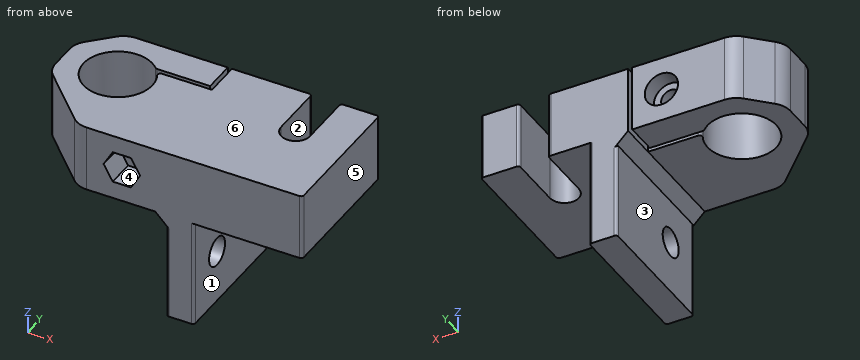
```python
from build123d import *

# Parameters (mm, degrees)
PAD_DEPTH       = 31.5
SKETCH001_W     = 20
SKETCH001_H     = 30
SKETCH001_W_2   = 27
POCKET_DEPTH    = 19.5
SKETCH002_R     = 2.6
POCKET001_DEPTH = 24.501
SKETCH003_R     = 1.7
POCKET002_DEPTH = 25.001
SKETCH004_R     = 3
POCKET003_DEPTH = 3
POCKET004_DEPTH = 5
CHAMFER_SIZE    = 2
FILLET_R        = 0.5


with BuildPart() as body:
    # Sketch → Pad (new body)
    with BuildSketch(Plane.XY):
        with BuildLine():
            ThreePointArc((-0.171573, -13.828427), (1.126121, -14.695518), (2.656854, -15))
            Line((41.00007, -14.999422), (2.656854, -15))
            ThreePointArc((41.00007, -14.999422), (41.353579, -14.85295), (41.5, -14.499421))
            Line((41.5, 9.5), (41.5, -14.499421))
            ThreePointArc((41.5, 9.5), (41.353578, 9.853528), (41.000071, 10))
            Line((34.6, 10), (41.000071, 10))
            Line((34.6, 10), (34.6, 0))
            ThreePointArc((29.4, 0), (32, -2.6), (34.6, 0))
            Line((29.4, 0), (29.4, 10))
            Line((15, 10), (29.4, 10))
            Line((15, 3.5), (15, 10))
            Line((5.990826, 3.5), (15, 3.5))
            ThreePointArc((5.990826, 3.5), (5.56542, 3.262735), (5.54375, 2.776119))
            ThreePointArc((4.372572, 4.395522), (-5.023841, -3.633322), (5.54375, 2.776119))
            ThreePointArc((4.372572, 4.395522), (4.534461, 4.28781), (4.725198, 4.25))
            Line((14.25, 4.25), (4.725198, 4.25))
            Line((14.25, 10), (14.25, 4.25))
            Line((-2.343146, 10), (14.25, 10))
            ThreePointArc((-2.343146, 10), (-3.873879, 9.695518), (-5.171573, 8.828427))
            Line((-5.171573, 8.828427), (-8.828427, 5.171573))
            ThreePointArc((-8.828427, 5.171573), (-9.695518, 3.873879), (-10, 2.343146))
            Line((-10, -2.343146), (-10, 2.343146))
            ThreePointArc((-10, -2.343146), (-9.695518, -3.873879), (-8.828427, -5.171573))
            Line((-8.828427, -5.171573), (-0.171573, -13.828427))
        make_face()
    extrude(amount=PAD_DEPTH)

    # Sketch001 (on Face26 of Pad) → Pocket (cut)
    with BuildSketch(Plane.XY.offset(31.5)):
        with Locations((32, 0)):
            Rectangle(SKETCH001_W, SKETCH001_H)
        with Locations((3.5, 0)):
            Rectangle(SKETCH001_W_2, SKETCH001_H)
    extrude(amount=-POCKET_DEPTH, mode=Mode.SUBTRACT)

    # Sketch002 (on Face29 of Pocket) → Pocket001 (cut, through all)
    with BuildSketch(Plane(origin=(17, 0, 0), x_dir=(0, -1, 0), z_dir=(-1, 0, 0))):
        with Locations((7.5, 22)):
            Circle(SKETCH002_R)
    extrude(amount=-POCKET001_DEPTH, mode=Mode.SUBTRACT)

    # Sketch003 (on Face13 of Pocket001) → Pocket002 (cut, through all)
    with BuildSketch(Plane(origin=(0, 10, 0), x_dir=(-1, 0, 0), z_dir=(0, 1, 0))):
        with Locations((-9, 6)):
            Circle(SKETCH003_R)
    extrude(amount=-POCKET002_DEPTH, mode=Mode.SUBTRACT)

    # Sketch004 (on Face13 of Pocket002) → Pocket003 (cut)
    with BuildSketch(Plane(origin=(0, 10, 0), x_dir=(-1, 0, 0), z_dir=(0, 1, 0))):
        with Locations((-9, 6)):
            Circle(SKETCH004_R)
    extrude(amount=-POCKET003_DEPTH, mode=Mode.SUBTRACT)

    # Sketch005 (on Face21 of Pocket003) → Pocket004 (cut)
    with BuildSketch(Plane(origin=(0.000226, -15.00004, 0), x_dir=(1, 1.5e-05, 0), z_dir=(1.5e-05, -1, 0))):
        Polygon((10.645448, 3.15), (12.290897, 6), (10.645448, 8.85), (7.354552, 8.85), (5.709103, 6), (7.354552, 3.15), align=None)
    extrude(amount=-POCKET004_DEPTH, mode=Mode.SUBTRACT)

    # Chamfer
    chamfer_edges = [body.edges().sort_by_distance(p)[0] for p in [
        (17, -2.499892, 12),
    ]]
    chamfer(chamfer_edges, length=CHAMFER_SIZE)

    # Fillet
    fillet_edges = [body.edges().sort_by_distance(p)[0] for p in [
        (34.6, 10, 6),
        (29.4, 10, 6),
        (22, 10, 21.75),
        (22, -14.999708, 21.75),
        (17, 10, 22.75),
        (17, -14.999784, 22.75),
    ]]
    fillet(fillet_edges, radius=FILLET_R)


with BuildPart() as part_mirroring:
    # Part__Mirroring: instance of Body
    add(body.part.mirror(Plane(origin=(15.75, -2.5, 0), x_dir=(0, 1, 0), z_dir=(0, 0, 1))))


solid = part_mirroring.part
```
The listing builds one solid part. Answer for the finished solid, in the listing's coordinates (mm). Face numbers are marked on the shaded views. A direction names the side the tool comes from. Round coordinates to 2 decimals unless told otherwise and drop trailing zeros. Order: outer loops, then holes, each group sorted by start corner. A loop starts at its lowest first (then second) coordinate and runs counter-clockwise, first axis right, second up. Notation, with made-up numbers: (-22.5, -3.5) - (3.5, -3.5) arc R26 ccw to (3.5, 26.5) - close; hole circle Ø7 at (-35, 61.5). An arc over 180 degrees is marked (long way). Put each result on its own line as item: value. Start each with the question number.
(1) Find section D-D (z = -28.5). Give the vertices of the cut face in (x, y), plus the area to 3 significant figures.
(2) Determine the mould class of the marked faces 4, 5 and 6 for opening direction Z: released by +Z, released by -Z, zero draft, split by the parting line, or undercut.
(3) Given P1, Ø7.5, axis at x = 0, y = 0, coming from the +Z side; P2, Ø10, axis at x = 9.5, z = -3.5, coming from the +Y side; P3, Ø6, axis at y = 2.5, z = -20.5, coming from the -X side; P4, Ø4.5, axis at x = 9, z = -6, coming from the +Y side, each flat-ended and moving along its own axis, determine where each tip first touches the part or whether it passes through.
(4) Find section C-C (x = 2). Give the vertices of the cut face in (y, z), plus the area to 3 significant figures.
(5) Straight lines are drawn through the part: probe 1 along Z at (x, y) = (9, -4.5); probe 2 along Z at (x, y) = (9, 9.2); probe 3 along X at (y, z) = (5.55, -6). For each, find the intervals that lie inside material, in ascending order. Write a range as from..to.
(6) Find section A-A (y = -7.5). Give the vertices of the cut face in (x, z), plus the area to 3 significant figures.
(7) Find section B-B (z = -22). Give the vertices of the cut face in (x, y), plus the area to 3 significant figures.
(8) For the marked faces 1, 2 and 3, determine the directions among +Z, -Z, +X, -X, +Y, -Y from which every point of the face is accessible in a straight line to the end or side of a thin tool.
Reply:
1. outline: (17, -14.5) arc R0.5 ccw to (17.5, -15) - (21.5, -15) arc R0.5 ccw to (22, -14.5) - (22, 9.5) arc R0.5 ccw to (21.5, 10) - (17.5, 10) arc R0.5 ccw to (17, 9.5) - close
1. area: 125 mm^2
2. face 4: undercut
2. face 5: zero draft
2. face 6: released by +Z
3. P1: through
3. P2: y = 10
3. P3: x = 17
3. P4: y = 7
4. outline: (-14.95, -12) - (-5.87, -12) - (-5.87, 0) - (-14.95, 0) - close; (5.87, -12) - (10, -12) - (10, 0) - (5.87, 0) - close
4. area: 159 mm^2
5. probe 1: -12..-7.7, -4.3..0
5. probe 2: -12..-9, -3..0
5. probe 3: -8.45..-2.76, 2.76..7.3, 10.7..14.25, 15..29.4, 34.6..41.5
6. outline: (-6.5, -12) - (15, -12) - (17, -14) - (17, -19.4) - (22, -19.4) - (22, -12) - (41.5, -12) - (41.5, 0) - (-6.5, 0) - close; (17, -31.5) - (22, -31.5) - (22, -24.6) - (17, -24.6) - close; hole circle Ø3.4 at (9, -6)
6. area: 640 mm^2
7. outline: (17, -14.5) arc R0.5 ccw to (17.5, -15) - (21.5, -15) arc R0.5 ccw to (22, -14.5) - (22, -10.1) - (17, -10.1) - close; (17, -4.9) - (22, -4.9) - (22, 9.5) arc R0.5 ccw to (21.5, 10) - (17.5, 10) arc R0.5 ccw to (17, 9.5) - close
7. area: 98.8 mm^2
8. face 1: -Z, +X, +Y, -Y
8. face 2: +Z, -Z, +Y
8. face 3: -Z, -X, +Y, -Y
